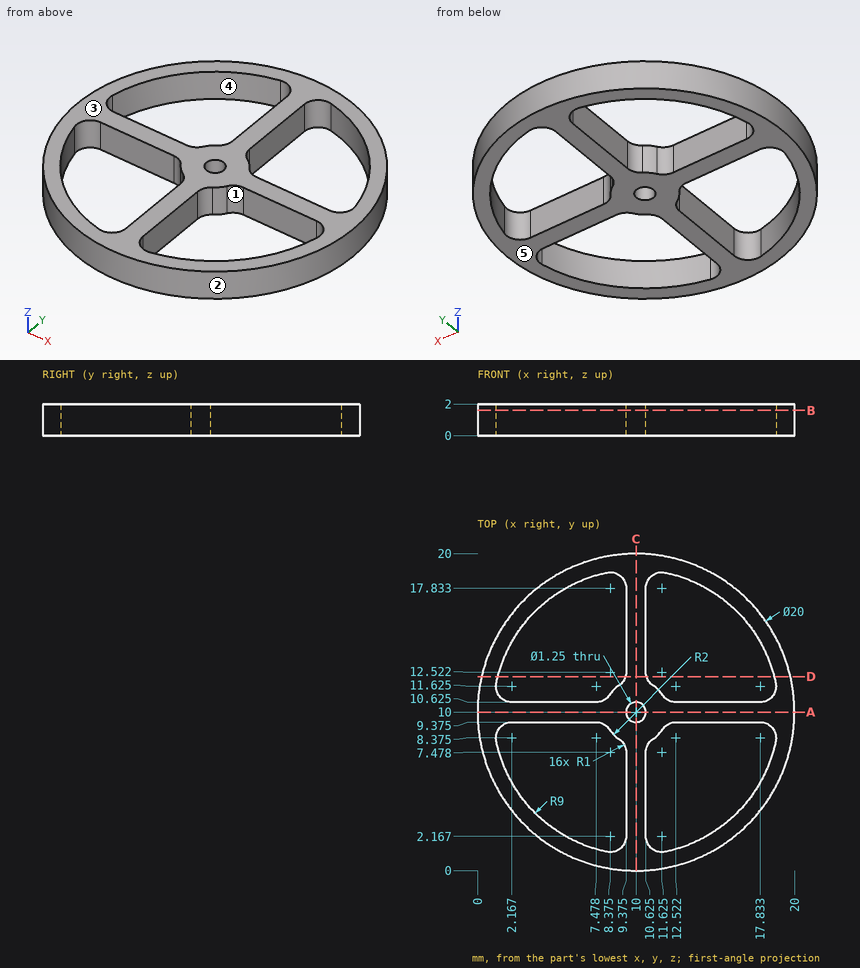
Verification items for this drawing (mm, ordinates from the low corner). A direction names the side the tool comes from. Give positions to 0.01 mm unless a question says otherwise; leave off trailing zeros. Loops run counter-clockwise (first coordinate to the right, second up) from the corner with the lowest first, then second, coordinate; pieces in that order, holes last.
(1) Release check for a two-part mould opening along X. For the marked faces 1, 2 and 3 record: released by +X, released by -X, zero draft, split by the parting line, or undercut.
From the geometry:
face 1: undercut
face 2: split by the parting line
face 3: zero draft
(2) Depth check by flat-ended pin: pin 1 Ø0.6 at (y, z) = (3.5, 0.5) entering from +X; pin 2 Ø1 at (y, z) = (14.5, 1.5) entering from -X (1 decimal); pin 3 Ø0.6 at (x, z) = (4, 1) entering from +Y. Enter the tip coordinate at first touch or a pass-through.
From the geometry:
pin 1: stops at x = 17.85
pin 2: stops at x = 0.8
pin 3: stops at y = 18.22
(3) Section check D-D on y = 12.25. Record the cut outline in (x, z).
From the geometry:
outline: (0.26, 0) - (1.29, 0) - (1.29, 2) - (0.26, 2) - close; (9.34, 0) - (10.66, 0) - (10.66, 2) - (9.34, 2) - close; (18.71, 0) - (19.74, 0) - (19.74, 2) - (18.71, 2) - close
(4) Set-up check for the marked faces 4 and 5: record each of +Z, -Z, +X, -X, +Y, -Y from which the full face is reachable in a straight line by a thin tool's end or side.
From the geometry:
face 4: +Z, -Z
face 5: -Z, +X, -X, +Y, -Y
(5) Section check A-A on y = 10. Record the cut outline in (x, z) (3 decimals), then the cut area to 3 significant figures.
From the geometry:
outline: (0, 0) - (9.375, 0) - (9.375, 2) - (0, 2) - close; (10.625, 0) - (20, 0) - (20, 2) - (10.625, 2) - close
area: 37.5 mm2
(6) Thickness scan on L1, parallel to Y at x = 17, z = 1.6 (1 decimal); L2, parallel to X at y = 18, z = 0.8 (1 decimal); L3, parallel to Y at x = 10, z = 1.6 (3 decimals). Record the ranges inside material, lowest first.
From the geometry:
L1: y = 2.9 to 4.3, 9.4 to 10.6, 15.7 to 17.1
L2: x = 4 to 5.9, 9.4 to 10.6, 14.1 to 16
L3: y = 0 to 9.375, 10.625 to 20
(7) Section check B-B on z = 1.6. Count the separate pieces of the cut face and the enclosed holes in it, then the cut area to 3 significant figures.
From the geometry:
separate pieces: 1
enclosed holes: 5
area: 109 mm2
